Build history of the part. All positions in model axes, mm. A direction names the side the tool comes from. Give positions to 0.01 mm unless a question says otherwise; leave off trailing zeros. Write each loop counter-clockwise with the first axis right and the second up, starting at its lowest first coordinate (ties: lowest second). Pieces come first, ordered by that corner, then holes. Notation, with made-up numbers: (23, 0.5) -> (29, 0.5) arc R21 cw to (29, 7.5) -> close; hole circle Ø1 at (15, 17.25). An arc over 180 degrees is marked (long way). One line per question, with ' | ' between items. Start each with the question number.
(1) Tool access for faces 1 (the flat face through (-35.5, -25, 5)), 2 (the flat face through (11, -29, 3.5)), 3 (the flat face through (-27.5, -25, 5)), 4 (the flat face through (27.5, 9, 12)): list every direction of +Z, -Z, +X, -X, +Y, -Y with a clear straight run to the whole face (end or side of a thin tool).
(2) Band-saw the part on C-C, the plane z = 5.25. Count the separate pieces of the cut face and the enclosed holes in it, and give its area (3 significant figures).
(3) Drill centre lines: probe 1 along Y at (x, z) = (-39.2, 0.7); probe 2 along X at (y, z) = (-24.7, 1.35); probe 3 along X at (y, z) = (23.5, 2.5). Where is each one in solid material? Low to high. Write a range as from..to.
(4) Pull direction Y, two halves, no side cores. Call faces 5 (the flat face through (44.5, -18, 10)), 6 (the cylindrical face through (19.87, -25.68, 1.77)), 7 (the flat face through (11, -30.6, 6)): released by +Y, released by -Y, zero draft, split by the parting line, or undercut.
(5) Band-saw the part on D-D, the plane z = 11. Give the cut face in (x, y), and give its area (3 significant figures).
(6) Band-saw the part on B-B, the plane y = 24.7. Give the cut face in (x, z), and give its area (3 significant figures).
(7) Band-saw the part on A-A, the plane x = -39.2. Give the cut face in (y, z).
(8) Pin check, flat tips, straight feed: P1, Ø8, axis at x = 15.5, y = -22.5, coming from the +Z side; P2, Ø8, axis at x = 1.5, y = -6, coming from the -Z side; P3, Ø1.9, axis at x = -11, z = 2, coming from the -Y side; P4, Ø3, axis at y = 0.5, z = 12, coming from the -X side. Stop position of each tip, or through.
from build123d import *

# Parameters (mm, degrees)
F0_W     = 85
F0_H     = 56
F1_DEPTH = 3.5
F2_W     = 50
F2_H     = 5
F3_DEPTH = 9.3
F2_W_2   = 4
F2_H_2   = 22.2
F4_DEPTH = 5.5
F2_W_3   = 8
F2_H_3   = 5.4
F5_DEPTH = 2.7
F2_W_4   = 15
F2_H_4   = 1.8
F2_H_5   = 8.2
F6_DEPTH = 6
F2_W_5   = 7
F2_H_6   = 2.6
F2_H_7   = 12.4
F7_DEPTH = 6
F2_H_8   = 33
F2_W_6   = 2.2
F8_DEPTH = 16.3
F2_W_7   = 19.2
F2_H_9   = 16
F2_W_8   = 2
F9_DEPTH = 13.5
F10_D    = 2.9


with BuildPart() as f1:
    # F0 (on Top) → F1 (new body)
    with BuildSketch(Plane.XY):
        Rectangle(F0_W, F0_H)
    extrude(amount=F1_DEPTH)

    # F2 (on face) → F3 (join)
    with BuildSketch(Plane.XY.offset(3.5)):
        with Locations((-10, 24.2)):
            Rectangle(F2_W, F2_H)
    extrude(amount=F3_DEPTH)

    # F2 (on face) → F4 (join)
    with BuildSketch(Plane.XY.offset(3.5)):
        with Locations((-38.5, -0.1)):
            Rectangle(F2_W_2, F2_H_2)
        with Locations((3.5, -16.1)):
            Rectangle(F2_W_2, F2_H_2)
    extrude(amount=F4_DEPTH)

    # F2 (on face) → F5 (join)
    with BuildSketch(Plane.XY.offset(3.5)):
        with Locations((-31.5, -25.3)):
            Rectangle(F2_W_3, F2_H_3)
    extrude(amount=F5_DEPTH)

    # F2 (on face) → F6 (join)
    with BuildSketch(Plane.XY.offset(3.5)):
        with Locations((-10, -28.9)):
            Rectangle(F2_W_4, F2_H_4)
        with Locations((-10, -23.9)):
            Rectangle(F2_W_4, F2_H_5)
    extrude(amount=F6_DEPTH)

    # F2 (on face) → F7 (join)
    with BuildSketch(Plane.XY.offset(3.5)):
        with Locations((11, -29.3)):
            Rectangle(F2_W_5, F2_H_6)
        with Locations((11, -21.8)):
            Rectangle(F2_W_5, F2_H_7)
    extrude(amount=F7_DEPTH)

    # F2 (on face) → F8 (join)
    with BuildSketch(Plane.XY.offset(3.5)):
        with Locations((35, 9.5)):
            Rectangle(F2_W_4, F2_H_8)
        with Locations((43.6, 9.5)):
            Rectangle(F2_W_6, F2_H_8)
    extrude(amount=F8_DEPTH)

    # F2 (on face) → F9 (join)
    with BuildSketch(Plane.XY.offset(3.5)):
        with Locations((32.9, -17.5)):
            Rectangle(F2_W_7, F2_H_9)
        with Locations((43.5, -17.5)):
            Rectangle(F2_W_8, F2_H_9)
    extrude(amount=F9_DEPTH)

    # F10 (through all)
    with Locations(Plane(origin=(0, 0, 0), x_dir=(1, 0, 0), z_dir=(0, 0, -1))):
        with Locations((18.8, 24.7), (-39.2, 24.7), (-39.2, -24.7), (18.8, -24.7)):
            Hole(F10_D / 2)


solid = f1.part
Results:
1) face 1: +Z, -X, +Y, -Y | face 2: -Z, +X, -X, -Y | face 3: +Z, -Y | face 4: +Z, +Y
2) separate pieces: 8 | enclosed holes: 0 | area: 1,630 mm²
3) probe 1: y = -28..-26.15, -23.25..23.25, 26.15..28 | probe 2: x = -42.5..-40.65, -37.75..17.35, 20.25..42.5 | probe 3: x = -42.5..-40.01, -38.39..17.99, 19.61..42.5
4) face 5: zero draft | face 6: undercut | face 7: released by -Y
5) outline: (-35, 21.7) -> (15, 21.7) -> (15, 26.7) -> (-35, 26.7) -> close; (23.3, -25.5) -> (44.5, -25.5) -> (44.5, -9.5) -> (23.3, -9.5) -> close; (27.5, -7) -> (44.7, -7) -> (44.7, 26) -> (27.5, 26) -> close | area: 1,160 mm²
6) outline: (-42.5, 0) -> (-40.65, 0) -> (-40.65, 3.5) -> (-42.5, 3.5) -> close; (-37.75, 0) -> (17.35, 0) -> (17.35, 3.5) -> (15, 3.5) -> (15, 12.8) -> (-35, 12.8) -> (-35, 3.5) -> (-37.75, 3.5) -> close; (20.25, 0) -> (42.5, 0) -> (42.5, 3.5) -> (44.7, 3.5) -> (44.7, 19.8) -> (27.5, 19.8) -> (27.5, 3.5) -> (20.25, 3.5) -> close | area: 1,020 mm²
7) outline: (-28, 0) -> (-26.15, 0) -> (-26.15, 3.5) -> (-28, 3.5) -> close; (-23.25, 0) -> (23.25, 0) -> (23.25, 3.5) -> (11, 3.5) -> (11, 9) -> (-11.2, 9) -> (-11.2, 3.5) -> (-23.25, 3.5) -> close; (26.15, 0) -> (28, 0) -> (28, 3.5) -> (26.15, 3.5) -> close
8) P1: stops at z = 9.5 | P2: stops at z = 0 | P3: stops at y = -28 | P4: stops at x = 27.5
